Geometry check sheet. Reference: drawing and pictorial views, mm from the part's lowest x, y, z. A direction names the side the tool comes from. Round coordinates to 2 decimals unless told otherwise and drop trailing zeros. Loops run counter-clockwise (first coordinate to the right, second up) from the corner with the lowest first, then second, coordinate; pieces in that order, holes last. Notation, with made-up numbers: (44, 45) - (95, 45) arc R16 ccw to (95, 61) - close; hole circle Ø9 at (18.5, 55). An arc over 180 degrees is marked (long way). Return JSON: item names as keys, results as strings.
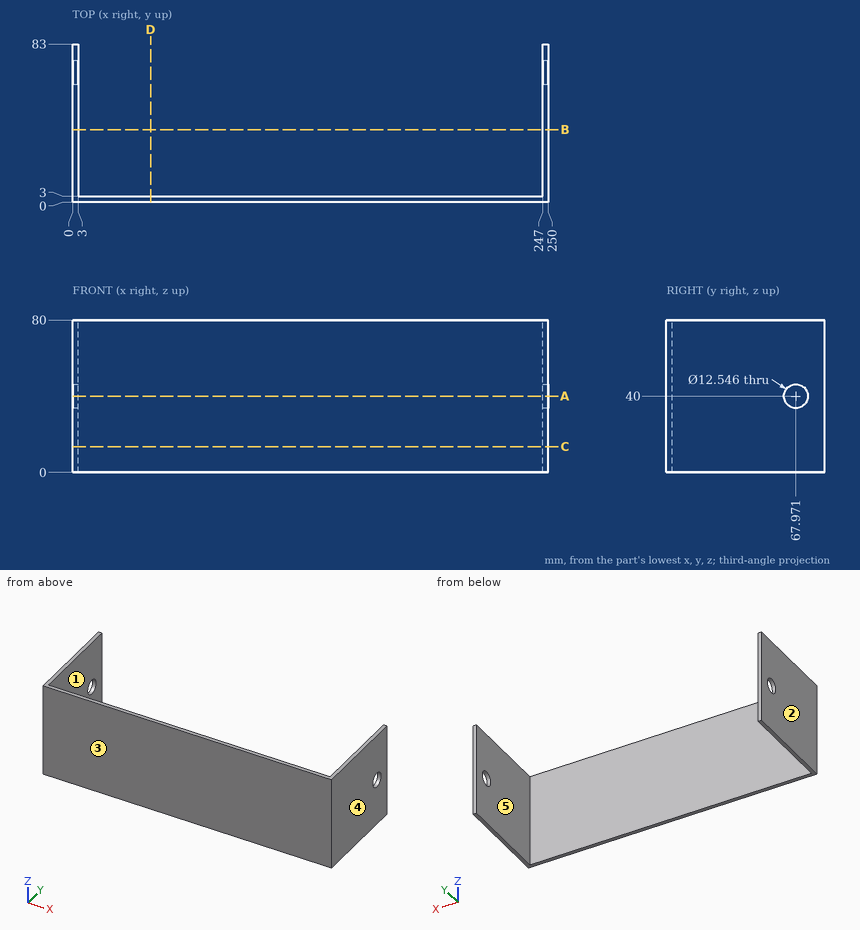
Q1. Sectioned sample at C-C (z = 13.5). Enter the section's corners in (x, y), plus the area to 3 significant figures.
Answer key:
{"outline": "(0, 0) - (250, 0) - (250, 83) - (247, 83) - (247, 3) - (3, 3) - (3, 83) - (0, 83) - close", "area": "1,230 mm²"}
Q2. Draft check along X on the marked faces 1, 2 and 3. Enter one of: released by +X, released by -X, zero draft, split by the parting line, or undercut.
Answer key:
{"face 1": "undercut", "face 2": "released by -X", "face 3": "zero draft"}
Q3. Depth check by flat-ended pin: P1, Ø1.5, axis at x = 119.5, z = 26.5, coming from the +Y side. Enter the tip coordinate at first touch or a pass-through.
Answer key:
{"P1": "stops at y = 3"}
Q4. Tool access check on the marked faces 4 and 5. Record the directions out of +Z, -Z, +X, -X, +Y, -Y that give a thin tool (end or side, any length) a straight path to the whole face; none if there is none.
Answer key:
{"face 4": "+Z, -Z, +X, +Y, -Y", "face 5": "+Z, -Z, +Y"}
Q5. Scan lines: probe 1 along Y at (x, z) = (1.2, 40); probe 2 along X at (y, z) = (76, 63); probe 3 along Y at (x, z) = (219.5, 58). Record each from-to range of solid material in increasing order. Write a range as [from, to].
Answer key:
{"probe 1": "y = [0, 61.7], [74.24, 83]", "probe 2": "x = [0, 3], [247, 250]", "probe 3": "y = [0, 3]"}
Q6. Sectioned sample at D-D (x = 41). Enter the section's corners in (y, z), plus the area to 3 significant figures.
Answer key:
{"outline": "(0, 0) - (3, 0) - (3, 80) - (0, 80) - close", "area": "240 mm²"}
Q7. Sectioned sample at B-B (y = 38). Enter the section's corners in (x, z), plus the area to 3 significant figures.
Answer key:
{"outline": "(0, 0) - (3, 0) - (3, 80) - (0, 80) - close; (247, 0) - (250, 0) - (250, 80) - (247, 80) - close", "area": "480 mm²"}
Q8. Sectioned sample at A-A (z = 40). Enter the section's corners in (x, y).
Answer key:
{"outline": "(0, 0) - (250, 0) - (250, 61.7) - (247, 61.7) - (247, 3) - (3, 3) - (3, 61.7) - (0, 61.7) - close; (0, 74.24) - (3, 74.24) - (3, 83) - (0, 83) - close; (247, 74.24) - (250, 74.24) - (250, 83) - (247, 83) - close"}
